from build123d import *

# Parameters (mm, degrees)
SKETCH1_R           = 26
BOSS_EXTRUDE1_DEPTH = 11
SKETCH2_R           = 21
CUT_EXTRUDE1_DEPTH  = 8
BOSS_EXTRUDE2_DEPTH = 8
SKETCH5_R           = 1
BOSS_EXTRUDE3_DEPTH = 8
SKETCH6_R           = 2.5
BOSS_EXTRUDE4_DEPTH = 8
SKETCH7_R           = 3.5
BOSS_EXTRUDE5_DEPTH = 8
SKETCH11_R          = 1.5
BOSS_EXTRUDE6_DEPTH = 8


with BuildPart() as part:
    # Sketch1 → Boss-Extrude1 (new body)
    with BuildSketch(Plane(origin=(0, 0, 0), x_dir=(1, 0, 0), z_dir=(0, 1, 0))):
        with Locations(Location((0, 0, 0), (0, 0, 270))):
            Circle(SKETCH1_R)
    extrude(amount=BOSS_EXTRUDE1_DEPTH)

    # Sketch2 → Cut-Extrude1 (cut)
    with BuildSketch(Plane(origin=(0, 11, 0), x_dir=(1, 0, 0), z_dir=(0, 1, 0))):
        with Locations(Location((0, 0, 0), (0, 0, 270))):
            Circle(SKETCH2_R)
    extrude(amount=-CUT_EXTRUDE1_DEPTH, mode=Mode.SUBTRACT)

    # Sketch3 → Boss-Extrude2 (add)
    with BuildSketch(Plane(origin=(0, 3, 0), x_dir=(1, 0, 0), z_dir=(0, 1, 0))):
        Polygon((0, 6.260990337), (-1.405679911, 1.934752416), (-5.954555658, 1.934752416), (-2.274437874, -0.739009663), (-3.680117785, -5.065247584), (0, -2.391485505), (3.680117785, -5.065247584), (2.274437874, -0.739009663), (5.954555658, 1.934752416), (1.405679911, 1.934752416), align=None)
    extrude(amount=BOSS_EXTRUDE2_DEPTH)

    # Sketch5 → Boss-Extrude3 (add)
    with BuildSketch(Plane(origin=(0, 3, 0), x_dir=(1, 0, 0), z_dir=(0, 1, 0))):
        with Locations(Location((-9.706719743, 11.435890513, 0), (0, 0, 270))):
            Circle(SKETCH5_R)
    extrude(amount=BOSS_EXTRUDE3_DEPTH)

    # Sketch6 → Boss-Extrude4 (add)
    with BuildSketch(Plane(origin=(0, 3, 0), x_dir=(1, 0, 0), z_dir=(0, 1, 0))):
        with Locations(Location((0, 15, 0), (0, 0, 270))):
            Circle(SKETCH6_R)
    extrude(amount=BOSS_EXTRUDE4_DEPTH)

    # Sketch7 → Boss-Extrude5 (add)
    with BuildSketch(Plane(origin=(0, 3, 0), x_dir=(1, 0, 0), z_dir=(0, 1, 0))):
        with Locations(Location((13, -2, 0), (0, 0, 270))):
            Circle(SKETCH7_R)
    extrude(amount=BOSS_EXTRUDE5_DEPTH)

    # Sketch11 → Boss-Extrude6 (add)
    with BuildSketch(Plane(origin=(0, 3, 0), x_dir=(1, 0, 0), z_dir=(0, 1, 0))):
        with Locations(Location((5.064482164, -14.119172086, 0), (0, 0, 270))):
            Circle(SKETCH11_R)
    extrude(amount=BOSS_EXTRUDE6_DEPTH)


solid = part.part
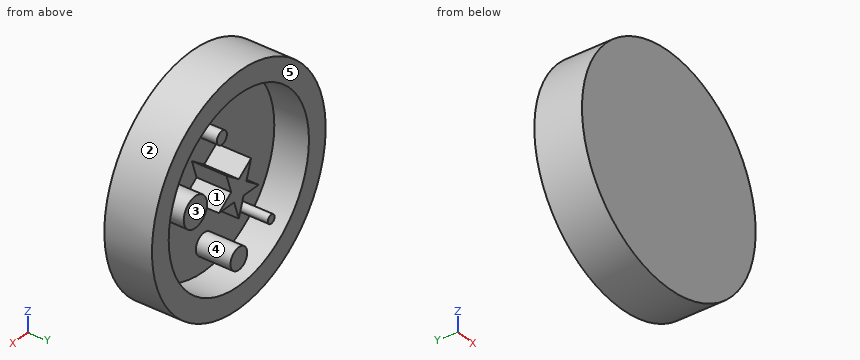
Check sheet for the modelled part. Datum: model origin and axes. Units: mm. Face numbers are marked on the shaded views. A direction names the side the tool comes from. Round coordinates to 2 decimals unless told otherwise and drop trailing zeros. Loops run counter-clockwise (first coordinate to the right, second up) from the corner with the lowest first, then second, coordinate; pieces in that order, holes last. Notation, with made-up numbers: (41, 88.5) -> (82, 88.5) arc R32 ccw to (82, 120.5) -> close; hole circle Ø2 at (76, -32). An arc over 180 degrees is marked (long way). Put each result on its own line as item: value. Start each with the question number.
1. Section check D-D (z = -16). Enter the section's corners in (x, y), plus the area to 3 significant figures.
2. Section check C-C (z = 10). Enter the section's corners in (x, y), plus the area to 3 significant figures.
3. Gauge pin test, flat ends, axial feed: pin 1 (4 mm diameter, centred on x = -13, y = 1, fed in from -Z); pin 2 (21 mm diameter, centred on x = -3, z = -6.5, fed in from +Y); pin 3 (4 mm diameter, centred on y = 8.5, z = 2, fed in from -X); pin 4 (2 mm diameter, centred on x = 2, y = 7.5, fed in from +Z). Record the tip position at first contact, or that the pin passes through.
4. Draft check along Z on the marked faces 1, 2 and 3. Enter one of: +Z half, -Z half, draft (parallel to the pull), parting line (faces both ways), or undercut.
5. Scan lines: probe 1 along X at (y, z) = (5.75, 0); probe 2 along X at (y, z) = (6.25, 2); probe 3 along Z at (x, y) = (-5, 6.5). Record each from-to range of solid material in increasing order.
6. Access from +Z, -Z, +X, -X, +Y, -Y to the whole of each face (thin tool, end or side, straight path). Record for the marked faces 4 and 5.
7. Section check A-A (y = 7.75). Enter the section's corners in (x, z).
8. Section check B-B (x = 15.5). Enter the section's corners in (y, z).
Findings:
1. outline: (-20.49, 0) -> (20.49, 0) -> (20.49, 11) -> (13.6, 11) -> (13.6, 3) -> (2.29, 3) -> (2.29, 11) -> (-2.29, 11) -> (-2.29, 3) -> (-13.6, 3) -> (-13.6, 11) -> (-20.49, 11) -> close
1. area: 270 mm^2
2. outline: (-24, 0) -> (24, 0) -> (24, 11) -> (18.47, 11) -> (18.47, 3) -> (-18.47, 3) -> (-18.47, 11) -> (-24, 11) -> close
2. area: 233 mm^2
3. pin 1: stops at z = -23.56
3. pin 2: stops at y = 11
3. pin 3: stops at x = -26
3. pin 4: stops at z = 25.98
4. face 1: undercut
4. face 2: parting line
4. face 3: draft
5. probe 1: x = -26 to -21, -3.29 to 3.29, 10.13 to 15.87, 21 to 26
5. probe 2: x = -25.92 to -20.9, -2.68 to 2.68, 9.5 to 16.5, 20.9 to 25.92
5. probe 3: z = -25.51 to -20.4, -1.93 to -1.24, 20.4 to 25.51
6. face 4: +Y
6. face 5: +Z, -Z, +X, -X, +Y
7. outline: circle Ø52 at (0, 0); circle Ø2 at (-9.71, -11.44); (-5.95, -1.93) -> (-1.41, -1.93) -> (0, -6.26) -> (1.41, -1.93) -> (5.95, -1.93) -> (2.27, 0.74) -> (3.68, 5.07) -> (0, 2.39) -> (-3.68, 5.07) -> (-2.27, 0.74) -> close; circle Ø5 at (0, -15); circle Ø3 at (5.06, 14.12); circle Ø7 at (13, 2); hole circle Ø42 at (0, 0)
8. outline: (0, -20.87) -> (11, -20.87) -> (11, -14.17) -> (3, -14.17) -> (3, -0.45) -> (11, -0.45) -> (11, 4.45) -> (3, 4.45) -> (3, 14.17) -> (11, 14.17) -> (11, 20.87) -> (0, 20.87) -> close
